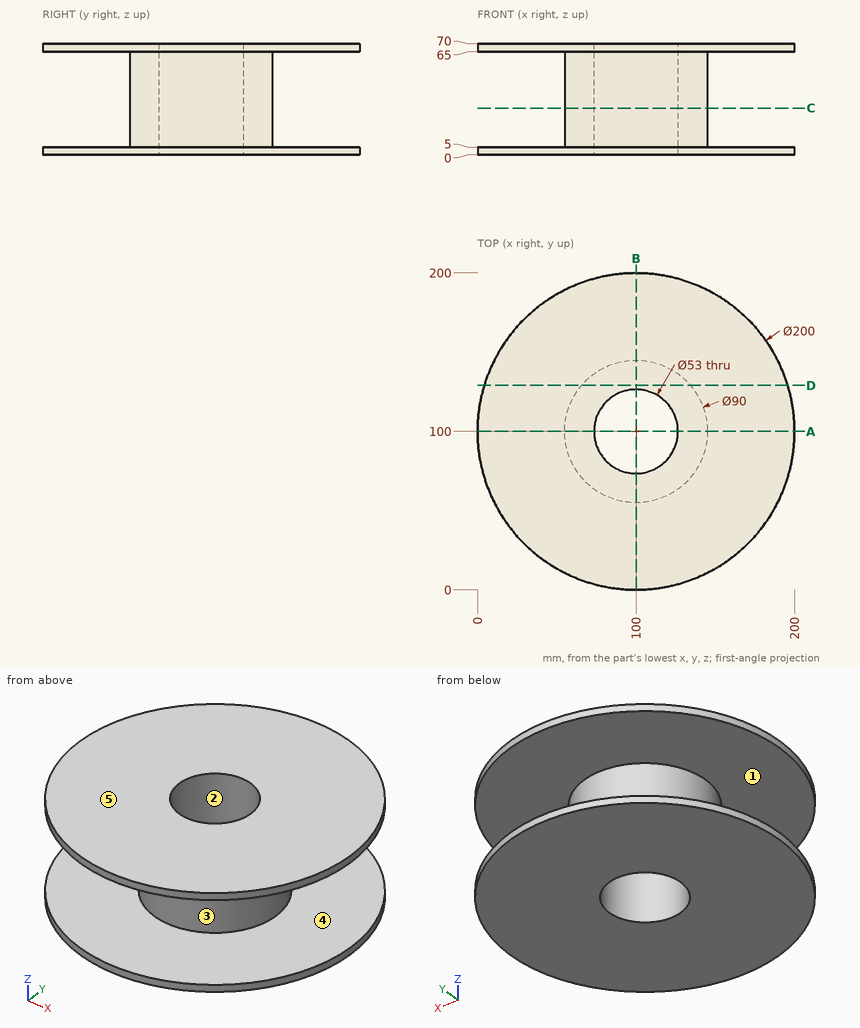
Part print with two shaded views. Sizes in mm from the minimum x, y, z corner. A direction names the side the tool comes from. Round coordinates to 2 decimals unless told otherwise and drop trailing zeros. Order: outer loops, then holes, each group sorted by start corner. A loop starts at its lowest first (then second) coordinate and runs counter-clockwise, first axis right, second up. Notation, with made-up numbers: M 57,85.25 L 76,85.25 A26 ccw 76,121.25 Z; hole C -19,15.25 d11. An arc over 180 degrees is marked long. Answer in a Markdown table with one row per item. Add a question column.
Q1. Cut at A-A on y = 100. Give the cut face in (x, z), and give its area (3 significant figures).
Q2. Pin check, flat tips, straight feed: pin 1 (1.5 mm diameter, centred on x = 85, z = 21.5, fed in from -Y); pin 2 (10 mm diameter, centred on x = 105.5, z = 58.5, fed in from -Y); pin 3 (3 mm diameter, centred on y = 100.5, z = 42.5, fed in from -X). Stop position of each tip, or through.
Q3. Cut at D-D on y = 129. Give the cut face in (x, z).
Q4. Mould opens along Y. For the marked faces 1, 2 and 3 say: +Y half, -Y half, draft (parallel to the pull), parting line (faces both ways), or undercut.
Q5. Wall check: L1, parallel to Z at x = 99, y = 40; L2, parallel to Y at x = 100, z = 33.5; L3, parallel to X at y = 81, z = 36. Give the ranges that are in metal, low to high. Write a range as from..to.
Q6. 3-axis set-ups, long thin cutter, end or side, ignore diameter. For the marked faces 4 and 5: which of +Z, -Z, +X, -X, +Y, -Y reach the whole face in a straight line?
Q7. Cut at C-C on z = 29.5. Give the cut face in (x, y), and give its area (3 significant figures).
Established:
| question | item | result |
|---|---|---|
| 1 | outline | M 0,0 L 73.5,0 L 73.5,70 L 0,70 L 0,65 L 55,65 L 55,5 L 0,5 Z; M 126.5,0 L 200,0 L 200,5 L 145,5 L 145,65 L 200,65 L 200,70 L 126.5,70 Z |
| 1 | area | 3,690 mm2 |
| 2 | pin 1 | stops at y = 57.32 |
| 2 | pin 2 | stops at y = 55 |
| 2 | pin 3 | stops at x = 55 |
| 3 | outline | M 4.3,0 L 195.7,0 L 195.7,5 L 134.41,5 L 134.41,65 L 195.7,65 L 195.7,70 L 4.3,70 L 4.3,65 L 65.59,65 L 65.59,5 L 4.3,5 Z |
| 4 | face 1 | draft |
| 4 | face 2 | undercut |
| 4 | face 3 | parting line |
| 5 | L1 | z = 0..5, 65..70 |
| 5 | L2 | y = 55..73.5, 126.5..145 |
| 5 | L3 | x = 59.21..81.53, 118.47..140.79 |
| 6 | face 4 | none |
| 6 | face 5 | +Z, +X, -X, +Y, -Y |
| 7 | outline | C 100,100 d90; hole C 100,100 d53 |
| 7 | area | 4,160 mm2 |
